```python
from build123d import *

# Parameters (mm, degrees)
F0_W     = 2.65
F0_H     = 18.9585
F2_SIZE2 = 1.5
F2_SIZE  = 1.5
F4_D     = 6.8
F4_DEPTH = 15.75
F4_TIP   = 2.0429261047
F5_SIZE2 = 2.5
F5_SIZE  = 2.5


with BuildPart() as f1:
    # F0 (on Right) → F1 (revolve)
    with BuildSketch(Plane.YZ):
        Polygon((-77.075, 13.8), (-77.075, 0), (25.925, 0), (25.925, 18.9585), (25.925, 20), (22.925, 20), (22.925, 13.8), align=None)
        with Locations((27.25, 9.47925)):
            Rectangle(F0_W, F0_H)
        Polygon((28.575, 18.9585), (28.575, 0), (77.075, 0), (77.075, 10), (92.075, 10), (92.075, 20), (28.575, 20), align=None)
    revolve(axis=Axis((0, 0, 0), (0, 1, 0)))

    # F2
    f2_edges = [f1.edges().sort_by_distance(p)[0] for p in [
        (0, 92.075, -10),
    ]]
    chamfer(f2_edges, length=F2_SIZE, length2=F2_SIZE2)

    # F4
    with Locations(Plane(origin=(0, 77.075, 0), x_dir=(-1, 0, 0), z_dir=(0, 1, 0))):
        with Locations((0, 0)):
            Hole(F4_D / 2, depth=F4_DEPTH)
            with Locations((0, 0, -(F4_DEPTH + F4_TIP / 2))):  # 118° drill point
                Cone(0, F4_D / 2, F4_TIP, mode=Mode.SUBTRACT)

    # F5
    f5_edges = [f1.edges().sort_by_distance(p)[0] for p in [
        (0, -77.075, -13.8),
    ]]
    chamfer(f5_edges, length=F5_SIZE, length2=F5_SIZE2)


solid = f1.part
```
Geometry check sheet. Reference: the model listing, model coordinates, mm. A direction names the side the tool comes from. Give positions to 0.01 mm unless a question says otherwise; leave off trailing zeros. Write each loop counter-clockwise with the first axis right and the second up, starting at its lowest first coordinate (ties: lowest second). Pieces come first, ordered by that corner, then holes. Notation, with made-up numbers: (-33, 47.5) -> (-14, 47.5) arc R16 ccw to (-14, 73.5) -> close; hole circle Ø4 at (13, 40.5). An arc over 180 degrees is marked (long way). Use one line per item in the form item = value.
Item 1: Mould release check, pull along X, two halves, no side actions. Record for faces 1 (the cylindrical face through (-9.76, 83.92, -2.17)), 2 (the flat face through (15, 25.925, -12)), 3 (the conical face through (-11.15, -76.95, -2.48)): released by +X, released by -X, zero draft, split by the parting line, or undercut.
Results list:
face_1 = undercut
face_2 = zero draft
face_3 = split by the parting line
Item 2: Access from +Z, -Z, +X, -X, +Y, -Y to the whole of each face (thin tool, end or side, straight path). Record for faces 4 (the cylindrical face through (-19.524, 59.881, -4.336)), 5 (the flat face through (15, 28.575, 12)), 6 (the flat face through (0, 77.075, -4)), 7 (the cylindrical face through (13.683, -26.507, -1.796)).
Results list:
face_4 = +Y, -Y
face_5 = none
face_6 = +Y
face_7 = -Y
Item 3: Depth check by flat-ended pin: pin 1 Ø1.5 at (y, z) = (32, -11.5) entering from +X; pin 2 Ø5 at (x, y) = (-8.5, 61.5) entering from +Z; pin 3 Ø1.5 at (x, y) = (2.5, -29) entering from -Z. Enter the tip coordinate at first touch or a pass-through.
Results list:
pin_1 = 16.87
pin_2 = 19.08
pin_3 = -13.69
Item 4: Sectioned sample at A-A on y = -31.5. Enter the section's corners in (x, z).
Results list:
outline = circle Ø27.6 at (0, 0)
Item 5: Scan lines: line 1 (X direction, y = 82.5, z = 0); line 2 (X direction, y = 69, z = 0); line 3 (Y direction, x = -4.5, z = 18.5) (3 decimals). Record each from-to range of solid material in increasing order.
Results list:
line_1 = -20 to -10, 10 to 20
line_2 = -20 to -3.4, 3.4 to 20
line_3 = 22.925 to 25.925, 28.575 to 92.075
